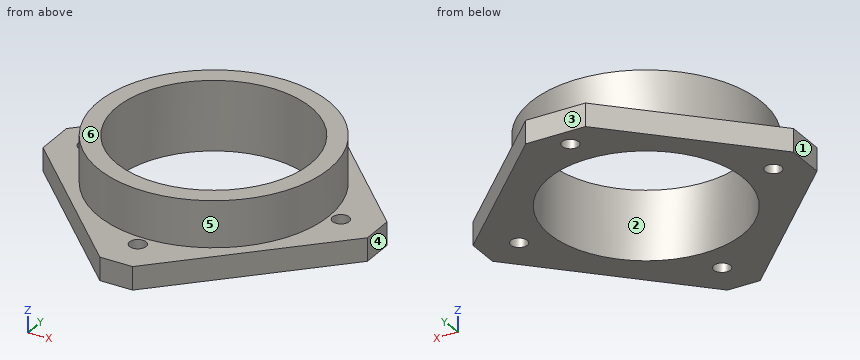
from build123d import *

# Parameters (mm, degrees)
SKETCH1_R           = 1.8
SKETCH1_R_2         = 21
BOSS_EXTRUDE1_DEPTH = 5
SKETCH2_R           = 25
SKETCH2_R_2         = 21
BOSS_EXTRUDE2_DEPTH = 10


with BuildPart() as part:
    # Sketch1 → Boss-Extrude1 (new body)
    with BuildSketch(Plane.XY):
        Polygon((-3.535533906, -35.355339059), (-34.029102601, -4.861770365), (-34.029102601, 3.62351101), (-5.832808457, 31.819805153), (7.071067812, 31.819805153), (35.355339059, 3.535533906), (35.355339059, -3.535533906), (3.535533906, -35.355339059), align=None)
        with Locations((27.5, 0)):
            Circle(SKETCH1_R, mode=Mode.SUBTRACT)
        with Locations((0, -27.5)):
            Circle(SKETCH1_R, mode=Mode.SUBTRACT)
        with Locations((0, 27.5)):
            Circle(SKETCH1_R, mode=Mode.SUBTRACT)
        Circle(SKETCH1_R_2, mode=Mode.SUBTRACT)
        with Locations((-27.5, 0)):
            Circle(SKETCH1_R, mode=Mode.SUBTRACT)
    extrude(amount=BOSS_EXTRUDE1_DEPTH)

    # Sketch2 → Boss-Extrude2 (add)
    with BuildSketch(Plane.XY.offset(5)):
        Circle(SKETCH2_R)
        Circle(SKETCH2_R_2, mode=Mode.SUBTRACT)
    extrude(amount=BOSS_EXTRUDE2_DEPTH)


solid = part.part
Work out the finished part from the listing and answer in its coordinate system (mm). Face numbers are marked on the shaded views. A direction names the side the tool comes from. Round coordinates to 2 decimals unless told otherwise and drop trailing zeros. Loops run counter-clockwise (first coordinate to the right, second up) from the corner with the lowest first, then second, coordinate; pieces in that order, holes last. Notation, with made-up numbers: M 3.25,-18 L 42.25,-18 A12 ccw 42.25,-10 Z; hole C 12.5,19 d6. An arc over 180 degrees is marked long. One line per question, with ' | ' between items. Start each with the question number.
(1) A tool of negligible diameter and unlimited length cuts with its end or side. For the marked faces 5 and 6, from which of +Z, -Z, +X, -X, +Y, -Y can it reach the whole face along a straight path? Write none if from no direction.
(2) A cutting plane is placed at B-B on y = 0. Write down the section's boundary in (x, z), plus the area to 3 significant figures.
(3) For a pull along X with two mould halves and no side action, classify the marked faces 1, 2, 3 and 4 as released by +X, released by -X, zero draft, split by the parting line, or undercut.
(4) A cutting plane is placed at C-C on z = 2.75. Write down the section's boundary in (x, y).
(5) Flat-ended cylindrical pins translate along their axes: pin 1 Ø4 at (x, z) = (-11, 13) entering from -Y; pin 2 Ø4.5 at (x, y) = (27.5, 0) entering from -Z; pin 3 Ø4 at (x, y) = (0, -27.5) entering from +Z; pin 4 Ø2 at (y, z) = (9, 8) entering from -X. Find the tip coordinate at first contact, or state that the pin passes through.
(6) A cutting plane is placed at D-D on y = 27.5. Write down the section's boundary in (x, z).
(7) Find the intervals of material crossed by line 1 (Y direction, x = 0, z = 2.2); line 2 (Y direction, x = 5, z = 1); line 3 (Y direction, x = 1.5, z = 10), in increasing order.
(8) A cutting plane is placed at A-A on x = 0. Write down the section's boundary in (y, z), plus the area to 3 significant figures.
Geometry check:
1) face 5: +Z | face 6: +Z, +X, -X, +Y, -Y
2) outline: M -34.03,0 L -29.3,0 L -29.3,5 L -34.03,5 Z; M -25.7,0 L -21,0 L -21,15 L -25,15 L -25,5 L -25.7,5 Z; M 21,0 L 25.7,0 L 25.7,5 L 25,5 L 25,15 L 21,15 Z; M 29.3,0 L 35.36,0 L 35.36,5 L 29.3,5 Z | area: 181 mm²
3) face 1: released by -X | face 2: undercut | face 3: zero draft | face 4: released by +X
4) outline: M -34.03,-4.86 L -3.54,-35.36 L 3.54,-35.36 L 35.36,-3.54 L 35.36,3.54 L 7.07,31.82 L -5.83,31.82 L -34.03,3.62 Z; hole C -27.5,0 d3.6; hole C 0,0 d42; hole C 0,-27.5 d3.6; hole C 0,27.5 d3.6; hole C 27.5,0 d3.6
5) pin 1: stops at y = -23.32 | pin 2: stops at z = 0 | pin 3: stops at z = 5 | pin 4: stops at x = -23.69
6) outline: M -10.15,0 L -1.8,0 L -1.8,5 L -10.15,5 Z; M 1.8,0 L 11.39,0 L 11.39,5 L 1.8,5 Z
7) line 1: y = -35.36 to -29.3, -25.7 to -21, 21 to 25.7, 29.3 to 31.82 | line 2: y = -33.89 to -20.4, 20.4 to 31.82 | line 3: y = -24.95 to -20.95, 20.95 to 24.95
8) outline: M -35.36,0 L -29.3,0 L -29.3,5 L -35.36,5 Z; M -25.7,0 L -21,0 L -21,15 L -25,15 L -25,5 L -25.7,5 Z; M 21,0 L 25.7,0 L 25.7,5 L 25,5 L 25,15 L 21,15 Z; M 29.3,0 L 31.82,0 L 31.82,5 L 29.3,5 Z | area: 170 mm²
